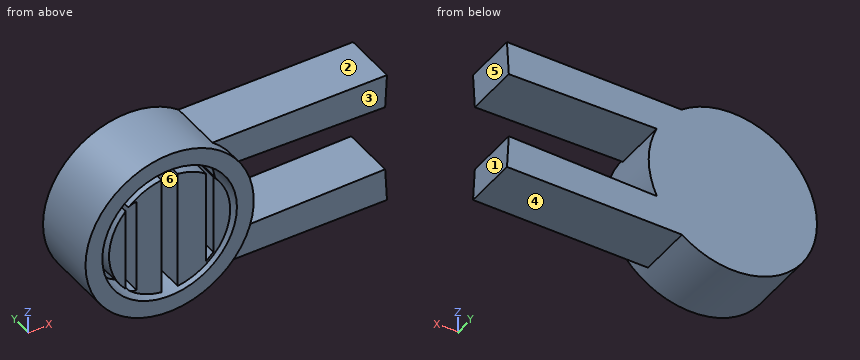
Autodesk Inventor part; units mm, degrees
ref_plane "YZ Plane" through (0, 0, 0) normal (1, 0, 0) x (0, 1, 0)
ref_plane "XZ Plane" through (0, 0, 0) normal (0, 1, 0) x (-1, 0, 0)
ref_plane "XY Plane" through (0, 0, 0) normal (0, 0, 1) x (1, 0, 0)
sketch "Sketch1" plane through (0, 0, 0) normal (0, 1, 0) x (-1, 0, 0)
  circle A0 centre (0, 0) radius 12.5
  circle A1 centre (0, 0) radius 10
  circle A2 centre (0, 0) radius 9
  dimension "d0" = 25
  dimension "d1" = 20
  dimension "d2" = 18
extrude "Extrusion1" add sketch "Sketch1" along normal blind 10 contours A0
sketch "Sketch2" plane through (0, 10, 0) normal (0, 1, 0) x (1, 0, 0)
  circle A0 centre (0, 0) radius 10
  circle A1 centre (0, 0) radius 9
  dimension "d5" = 18
extrude "Extrusion2" add sketch "Sketch2" against normal blind 10 contours A0 | A1
sketch "Sketch3" plane through (0, 0, 0) normal (0, -1, 0) x (1, 0, 0)
  circle A0 centre (0, 0) radius 10
  circle A1 centre (0, 0) radius 9
  dimension "d8" = 20
  dimension "d9" = 18
extrude "Extrusion3" cut sketch "Sketch3" against normal blind 5
sketch "Sketch4" plane through (0, 0, 0) normal (0, -1, 0) x (1, 0, 0)
  circle A0 centre (0, 0) radius 9
  line L0 (-6.5324, -6.191) -> (-6.5324, 6.191)
  line L1 (-4.9332, -7.0348) -> (-4.9332, 6.9906)
  arc A1 (-4.9332, 6.9906) -> (-6.5324, 6.191) centre (-4.9332, 4.9917) ccw
  arc A2 (-6.5324, -6.191) -> (-4.9332, -7.0348) centre (-4.9332, -5.0977) ccw
  point P0 (-6.1136, 6.6049)
  point P1 (-5.9735, -6.7318)
extrude "Extrusion4" cut sketch "Sketch4" against normal blind 5 contours A0 A1 L1 A2 L0
sketch "Sketch5" plane through (0, 0, 0) normal (0, -1, 0) x (1, 0, 0)
  arc A0 (-5.9735, -6.7318) -> (-6.1136, 6.6049) centre (0, 0) ccw
  line L0 (-1.1999, -8.9197) -> (-1.1999, 8.9197)
  line L1 (1.1999, 8.9197) -> (1.1999, -8.9197)
  line L2 (6.5028, 6.222) -> (6.5028, -5.7075)
  line L3 (6.5028, -5.7075) -> (5.4199, -6.7318)
  line L4 (5.4199, -6.7318) -> (5.4199, 7.185)
extrude "Extrusion5" cut sketch "Sketch5" against normal blind 5 contours L0 A0 L1 | L2 L3 L4 A0
sketch "Sketch6" plane through (0, 10, 0) normal (0, 1, 0) x (1, 0, 0)
  circle A0 centre (0, 0) radius 12.5
  line L0 (7.5517, 9.961) -> (33.5517, 9.961)
  line L1 (33.5517, 9.961) -> (33.2795, 4.9684)
  line L2 (33.2795, 4.9684) -> (11.2795, 5.3874)
  line L3 (13.1769, 0.0291) -> (33.0118, 0.0291)
  line L4 (7.5517, -9.9028) -> (33.5517, -9.9028)
  line L5 (33.5517, -9.9028) -> (33.2795, -4.9102)
  line L6 (33.2795, -4.9102) -> (11.2795, -5.3291)
  point P0 (11.3073, -5.3286)
  point P1 (7.6279, -9.9028)
  dimension "d16" = 26
  dimension "d17" = 5
  dimension "d18" = 22
extrude "Extrusion6" add sketch "Sketch6" against normal blind 8 contours A0 L0 L1 L2 | L6 L5 L4 A0
properties part number "ab"
Can you work these out from the model? Positions are in its coordinate system, mm. Face numbers are marked on the shaded views. A direction names the side the tool comes from. Coordinates: 2 decimals unless noted, no trailing zeros. Write each loop counter-clockwise with the first axis right and the second up, starting at its lowest first coordinate (ties: lowest second). Pieces come first, ordered by that corner, then holes. Notation, with made-up numbers: (-9.5, 73.25) - (37.5, 73.25) arc R11 ccw to (37.5, 88.25) - close; hole circle Ø2 at (63.5, 62.25). An arc over 180 degrees is marked (long way). Return JSON: item names as keys, results as strings.
Q1. If we section it at A-A (y = 8): Please give me the cut outline in (x, z), then the cut area to 3 significant figures.
Computed values:
{"outline": "(7.55, -9.96) - (33.55, -9.96) - (33.28, -4.97) - (11.28, -5.39) arc R12.5 ccw to (11.31, 5.33) - (33.28, 4.91) - (33.55, 9.9) - (7.63, 9.9) arc R12.5 ccw (long way) to start", "area": "717 mm2"}
Q2. If we section it at D-D (x = 27.5): Please give me the cut outline in (y, z).
Computed values:
{"outline": "(2, -9.96) - (10, -9.96) - (10, -5.08) - (2, -5.08) - close; (2, 5.02) - (10, 5.02) - (10, 9.9) - (2, 9.9) - close"}
Q3. Please list where these lines run through material, in increasing order: L1, parallel to Z at x = 0, y = 3.1; L2, parallel to Z at x = 25, y = 6; L3, parallel to Z at x = 9, y = 8.75. Write a range as from..to.
Computed values:
{"L1": "z = -12.5..-10, 10..12.5", "L2": "z = -9.96..-5.13, 5.07..9.9", "L3": "z = -9.96..9.9"}
Q4. I'm going to push flat-ended pins straight in: pin 1 Ø4 at (y, z) = (2, -1.5) entering from +X; pin 2 Ø5.5 at (y, z) = (3.5, -1) entering from -X; pin 3 Ø5.5 at (y, z) = (3, -2.5) entering from +X; pin 4 Ø2.5 at (x, y) = (24, 5) entering from +Z. Where does each tip first touch, or does it pass through?
Computed values:
{"pin 1": "stops at x = 12.5", "pin 2": "stops at x = -12.5", "pin 3": "stops at x = 33.29", "pin 4": "stops at z = 9.9"}
Q5. If we section it at C-C (y = 4): Please give me the cut outline in (x, z) (1 decimal).
Computed values:
{"outline": "(-6.5, -6.2) - (-6.5, 6.2) arc R9 ccw to start; (-6.1, 6.6) arc R2 cw to (-4.9, 7) - (-4.9, -7) arc R1.9 cw to (-6, -6.7) arc R9 ccw to (-1.2, -8.9) - (-1.2, 8.9) arc R9 ccw to start; (1.2, -8.9) arc R9 ccw to (6.5, 6.2) - (6.5, -5.7) - (5.4, -6.7) - (5.4, 7.2) arc R9 ccw to (1.2, 8.9) - close; (7.6, -10) - (33.6, -10) - (33.3, -5) - (11.3, -5.4) arc R12.5 ccw to (11.3, 5.3) - (33.3, 4.9) - (33.6, 9.9) - (7.6, 9.9) arc R12.5 ccw (long way) to start; hole circle Ø20 at (0, 0)"}
Q6. If we section it at B-B (z = 0): Please give me the cut outline in (x, y).
Computed values:
{"outline": "(-12.5, 0) - (-10, 0) - (-10, 5) - (-9, 5) - (-9, 0) - (-6.53, 0) - (-6.53, 5) - (-4.93, 5) - (-4.93, 0) - (-1.2, 0) - (-1.2, 5) - (1.2, 5) - (1.2, 0) - (5.42, 0) - (5.42, 5) - (6.5, 5) - (6.5, 0) - (9, 0) - (9, 5) - (10, 5) - (10, 0) - (12.5, 0) - (12.5, 10) - (-12.5, 10) - close"}
Q7. Thinking about a two-plate mould opening in X: for the marked faces 4, 5 and 6, which applies, +X half, -X half, draft (parallel to the pull), parting line (faces both ways), or undercut?
Computed values:
{"face 4": "draft", "face 5": "+X half", "face 6": "undercut"}
Q8. On a 3-axis mill with a long thin cutter (end or side, diameter ignored), from which of +Z, -Z, +X, -X, +Y, -Y can I reach the whole of each face in a straight line? I mean the marked faces 1, 2 and 3. Say none if no direction works.
Computed values:
{"face 1": "+X, +Y, -Y", "face 2": "+Z, +X, +Y, -Y", "face 3": "+Z, +X, -Y"}
